from build123d import *

# Parameters (mm, degrees)
BOSS_EXTRUDE1_DEPTH = 5.4
SKETCH2_R           = 2.5
BOSS_EXTRUDE2_DEPTH = 1.9
SKETCH3_W           = 12.4
SKETCH3_H           = 6.7
BOSS_EXTRUDE3_DEPTH = 0.2


with BuildPart() as part:
    # Sketch1 → Boss-Extrude1 (new body)
    with BuildSketch(Plane(origin=(0, 0, 0), x_dir=(1, 0, 0), z_dir=(0, 1, 0))):
        with BuildLine():
            Line((0, -3.15), (0, 3.15))
            Line((0, 3.15), (7.5, 3.15))
            Line((7.5, 3.15), (7.5, 3.6))
            ThreePointArc((7.5, 3.6), (8.1, 4.2), (8.7, 3.6))
            Line((8.7, 3.6), (8.7, 3.15))
            Line((8.7, 3.15), (12.4, 3.15))
            Line((12.4, 3.15), (12.4, -3.15))
            Line((12.4, -3.15), (8.7, -3.15))
            Line((8.7, -3.15), (8.7, -3.6))
            ThreePointArc((8.7, -3.6), (8.1, -4.2), (7.5, -3.6))
            Line((7.5, -3.6), (7.5, -3.15))
            Line((7.5, -3.15), (0, -3.15))
        make_face()
    extrude(amount=BOSS_EXTRUDE1_DEPTH)

    # Sketch2 → Boss-Extrude2 (add)
    with BuildSketch(Plane.ZY):
        with Locations(Location((0, 2.2, 0), (0, 0, 241.642363424))):  # turned: the seam where the file's is
            Circle(SKETCH2_R)
    extrude(amount=BOSS_EXTRUDE2_DEPTH)

    # Sketch3 → Boss-Extrude3 (add)
    with BuildSketch(Plane(origin=(0, 3.6, 0), x_dir=(-1, 0, 0), z_dir=(0, -1, 0))):
        with Locations((-6.2, 0)):
            Rectangle(SKETCH3_W, SKETCH3_H)
    extrude(amount=-BOSS_EXTRUDE3_DEPTH)


solid = part.part
Design review of the part built by this model. Coordinates are the model's own, in mm. A direction names the side the tool comes from. Round coordinates to 2 decimals unless told otherwise and drop trailing zeros. Loops run counter-clockwise (first coordinate to the right, second up) from the corner with the lowest first, then second, coordinate; pieces in that order, holes last. Notation, with made-up numbers: M 15,41.5 L 23,41.5 A22 ccw 23,49.5 Z; hole C 40,60.5 d4. An arc over 180 degrees is marked long. Answer as a JSON object with one key per item and string values.
Item 1: Machinability: for faces 1 (the flat face through (4, 2, -3.15)), 2 (the flat face through (11, 5, -3.15)), 3 (the flat face through (11, 2, -3.15)), 4 (the cylindrical face through (-0.937, 4.668, -0.396)), 5 (the flat face through (4, 5, 3.15)), which of the approach directions +Z, -Z, +X, -X, +Y, -Y give a long, thin tool a straight path to every point of the face, cutting with its end or side? Answer none if there is none.
Answer sheet:
{"face 1": "-Z, -X, -Y", "face 2": "-Z, +X, +Y", "face 3": "-Z, +X, -Y", "face 4": "-X", "face 5": "+Z, -X, +Y"}
Item 2: Wall thickness on L1, parallel to Z at x = 6.5, y = 2.65; L2, parallel to Y at x = 8.75, z = 2.5; L3, parallel to X at y = 2.2, z = -3: over which ranges is each line inside the solid? List them lowest first. Write a range as from..to.
Answer sheet:
{"L1": "z = -3.15..3.15", "L2": "y = 0..5.4", "L3": "x = 0..12.4"}
Item 3: We need section A-A on z = -1.5. Give the boundary of the cut face in (x, y).
Answer sheet:
{"outline": "M -1.9,0.2 L 0,0.2 L 0,0 L 12.4,0 L 12.4,5.4 L 0,5.4 L 0,4.2 L -1.9,4.2 Z"}
Item 4: We need section C-C on x = 3.75. Give the boundary of the cut face in (y, z).
Answer sheet:
{"outline": "M 0,-3.15 L 3.6,-3.15 L 3.6,-3.35 L 3.8,-3.35 L 3.8,-3.15 L 5.4,-3.15 L 5.4,3.15 L 3.8,3.15 L 3.8,3.35 L 3.6,3.35 L 3.6,3.15 L 0,3.15 Z"}
Item 5: We need section B-B on y = 2.2. Give the boundary of the cut face in (x, z), and give its area (3 significant figures).
Answer sheet:
{"outline": "M -1.9,-2.5 L 0,-2.5 L 0,-3.15 L 7.5,-3.15 L 7.5,-3.6 A0.6 ccw 8.7,-3.6 L 8.7,-3.15 L 12.4,-3.15 L 12.4,3.15 L 8.7,3.15 L 8.7,3.6 A0.6 ccw 7.5,3.6 L 7.5,3.15 L 0,3.15 L 0,2.5 L -1.9,2.5 Z", "area": "89.8 mm^2"}
Item 6: We need section D-D on y = 4.45. Give the boundary of the cut face in (x, z).
Answer sheet:
{"outline": "M -1.9,-1.09 L 0,-1.09 L 0,-3.15 L 7.5,-3.15 L 7.5,-3.6 A0.6 ccw 8.7,-3.6 L 8.7,-3.15 L 12.4,-3.15 L 12.4,3.15 L 8.7,3.15 L 8.7,3.6 A0.6 ccw 7.5,3.6 L 7.5,3.15 L 0,3.15 L 0,1.09 L -1.9,1.09 Z"}
Item 7: Clearance check with flat-ended pins moving along their axes: P1, Ø1, axis at x = 6.5, y = 4, coming from the +Z side; P2, Ø0.5, axis at x = 5, y = 4.5, coming from the +Z side; P3, Ø3, axis at x = 10, y = 2.5, coming from the -Z side. State where each tip first meets the part, or that it passes through.
Answer sheet:
{"P1": "stops at z = 3.35", "P2": "stops at z = 3.15", "P3": "stops at z = -4.05"}
